Read the model definition and answer for the solid it produces. Units are mm, in the model's axes. Round coordinates to 2 decimals unless told otherwise and drop trailing zeros. Loops run counter-clockwise (first coordinate to the right, second up) from the corner with the lowest first, then second, coordinate; pieces in that order, holes last. Notation, with made-up numbers: M -5.5,16.5 L 16.5,16.5 A9 cw 16.5,24.5 Z; hole C 55,74.25 d7. An arc over 180 degrees is marked long. Write each question's results on one line, items separated by ' | '.
```python
from build123d import *

# Parameters (mm, degrees)
BOSS_EXTRUDE1_DEPTH = 300
FILLET2_R           = 1


with BuildPart() as part:
    # Sketch1 → Boss-Extrude1 (new body)
    with BuildSketch(Plane.XY):
        Polygon((0, 0), (-20, 0), (-20, 5), (-15, 5), (-15, 4), (-18, 4), (-18, 1), (-2, 1), (-2, 4), (-5, 4), (-5, 5), (0, 5), align=None)
    extrude(amount=BOSS_EXTRUDE1_DEPTH)

    # Fillet2
    fillet2_edges = [part.edges().sort_by_distance(p)[0] for p in [
        (-18, 4, 150),
        (-2, 4, 150),
        (-2, 1, 150),
        (-18, 1, 150),
        (-20, 0, 150),
        (-20, 5, 150),
        (-15, 5, 150),
        (0, 0, 150),
        (0, 5, 150),
        (-5, 5, 150),
    ]]
    fillet(fillet2_edges, radius=FILLET2_R - 0.0001)  # a hair under: the kernel refuses the full size


solid = part.part
```
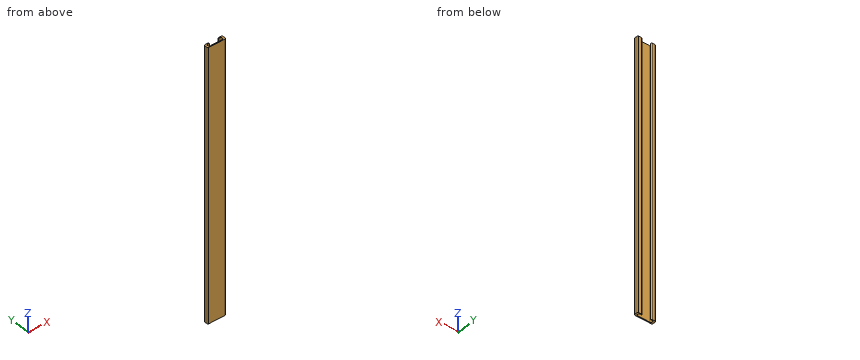
1. Find the intervals of material crossed by L1, parallel to X at y = 1.7, z = 248; L2, parallel to Y at x = -17, z = 195.5; L3, parallel to Y at x = -9.25, z = 107.5, in increasing order.
Completed:
L1: x = -20 to -17.95, -2.05 to 0 | L2: y = 0 to 1, 4 to 5 | L3: y = 0 to 1
2. Find section B-B, the plane x = -9. Give the vertices of the cut face in (y, z), then the cut area to 3 significant figures.
Completed:
outline: M 0,0 L 1,0 L 1,300 L 0,300 Z | area: 300 mm2
3. Given P1, Ø4, axis at x = -12.5, z = 173.5, coming from the +Y side; P2, Ø2, axis at x = -4.5, z = 39.5, coming from the +Y side, each flat-ended and moving along its own axis, determine where each tip first touches the part or whether it passes through.
Completed:
P1: stops at y = 1 | P2: stops at y = 5
